Geometry check sheet. Reference: the model listing, model coordinates, mm. Give positions to 0.01 mm unless a question says otherwise; leave off trailing zeros. Loops run counter-clockwise (first coordinate to the right, second up) from the corner with the lowest first, then second, coordinate; pieces in that order, holes last.
1. Release check for a two-part mould opening along Z. For faces 1 (the flat face through (-1, -2, -6)), 2 (the flat face through (12.167, -0.986, 53.67)), 3 (the flat face through (-12.12, -0.99, 53.75)), 4 (the cylindrical face through (34.82, -0.99, 40.02)) record: +Z half, -Z half, draft (parallel to the pull), parting line (faces both ways), or undercut.
2. Cross-section at C-C, the plane z = 15. Record the cut outline in (x, y), plus the area to 3 significant figures.
3. Material ranges on L1, parallel to Z at x = 0, y = -1.05; L2, parallel to X at y = -1.1, z = -0.5; L3, parallel to X at y = -0.35, z = -10, recorded low to high.
4. Go/stop test with flat-tipped pins: pin 1 Ø0.6 at (x, y) = (-67, -1.5) entering from -Z; pin 2 Ø1 at (x, y) = (-25, -0.5) entering from +Z. Record where each tip stops, or that it passes through.
5. Cross-section at A-A, the plane y = -1.3. Record the cut outline in (x, z).
6. Cross-section at B-B, the plane x = 14. Record the cut outline in (y, z).
from build123d import *

# Parameters (mm, degrees)
F1_DEPTH = 2


# Not quite as in the source:
# - a feature names something its author has since deleted; it is built from what else it names


with BuildPart() as f1:
    # F0 (on Front) → F1 (new body)
    with BuildSketch(Plane.XZ):
        with BuildLine():
            ThreePointArc((19.4604751144, -49.3491610835), (25.0909627965, -46.7385641336), (30.3780152375, -43.4882280802))
            ThreePointArc((30.3780152375, -43.4882280802), (47.0400422182, -24.5210974354), (53.0476181494, 0))
            Line((53.0476181494, 0), (-53.0476181494, 0))
            ThreePointArc((-53.0476181494, 0), (-43.8541995948, -29.8472606654), (-19.4604751144, -49.3491610835))
            ThreePointArc((-19.4604751144, -49.3491610835), (-6.4361640705, -14.8511496358), (23.054123582, -36.9886383414))
            ThreePointArc((23.054123582, -36.9886383414), (22.1374887057, -43.4248024119), (19.4604751144, -49.3491610835))
        make_face()
        with BuildLine():
            Line((-53.0476181494, 0), (53.0476181494, 0))
            ThreePointArc((53.0476181494, 0), (51.7146557328, 11.817113597), (47.7827569309, 23.0403544115))
            Line((47.7827569309, 23.0403544115), (15.6281781272, 50.6932918615))
            ThreePointArc((15.6281781272, 50.6932918615), (9.002371997, 52.2781702984), (2.2280864718, 53.0008058618))
            ThreePointArc((2.2280864718, 53.0008058618), (0, 52.7800319348), (-2.2280864718, 53.0008058618))
            ThreePointArc((-2.2280864718, 53.0008058618), (-9.0528372764, 52.2694550246), (-15.7260278086, 50.6630224196))
            Line((-15.7260278086, 50.6630224196), (-47.6465335474, 23.3207553961))
            ThreePointArc((-47.6465335474, 23.3207553961), (-51.6797102792, 11.9690156981), (-53.0476181494, 0))
        make_face()
        with BuildLine():
            ThreePointArc((47.7827569309, 23.0403544115), (51.7146557328, 11.817113597), (53.0476181494, 0))
            Line((53.0476181494, 0), (74.573867023, 0))
            Line((74.573867023, 0), (47.7827569309, 23.0403544115))
        make_face()
        with BuildLine():
            ThreePointArc((-19.4604751144, -49.3491610835), (0, -60.0427619235), (19.4604751144, -49.3491610835))
            ThreePointArc((19.4604751144, -49.3491610835), (0, -53.0476181494), (-19.4604751144, -49.3491610835))
        make_face()
        with BuildLine():
            ThreePointArc((-19.4604751144, -49.3491610835), (0, -53.0476181494), (19.4604751144, -49.3491610835))
            ThreePointArc((19.4604751144, -49.3491610835), (22.1374887057, -43.4248024119), (23.054123582, -36.9886383414))
            ThreePointArc((23.054123582, -36.9886383414), (-6.4361640705, -14.8511496358), (-19.4604751144, -49.3491610835))
        make_face()
        with BuildLine():
            Line((15.6281781272, 50.6932918615), (47.7827569309, 23.0403544115))
            ThreePointArc((47.7827569309, 23.0403544115), (34.5891299202, 40.2199189791), (15.6281781272, 50.6932918615))
        make_face()
        with BuildLine():
            Line((-74.8721584678, 0), (-53.0476181494, 0))
            ThreePointArc((-53.0476181494, 0), (-51.6797102792, 11.9690156981), (-47.6465335474, 23.3207553961))
            Line((-47.6465335474, 23.3207553961), (-74.8721584678, 0))
        make_face()
        with BuildLine():
            ThreePointArc((2.2280864718, 53.0008058618), (9.002371997, 52.2781702984), (15.6281781272, 50.6932918615))
            Line((15.6281781272, 50.6932918615), (8.6080503312, 56.7306016959))
            ThreePointArc((8.6080503312, 56.7306016959), (5.730035728, 54.3320712807), (2.2280864718, 53.0008058618))
        make_face()
        with BuildLine():
            ThreePointArc((-15.7260278086, 50.6630224196), (-34.5097127589, 40.2880815704), (-47.6465335474, 23.3207553961))
            Line((-47.6465335474, 23.3207553961), (-15.7260278086, 50.6630224196))
        make_face()
        with BuildLine():
            ThreePointArc((-2.2280864718, 53.0008058618), (0, 53.0476181494), (2.2280864718, 53.0008058618))
            ThreePointArc((2.2280864718, 53.0008058618), (5.730035728, 54.3320712807), (8.6080503312, 56.7306016959))
            Line((8.6080503312, 56.7306016959), (0, 64.1335248947))
            Line((0, 64.1335248947), (-8.6226387996, 56.7475989187))
            ThreePointArc((-8.6226387996, 56.7475989187), (-5.7397015847, 54.3377284437), (-2.2280864718, 53.0008058618))
        make_face()
        with BuildLine():
            Line((0, 64.1335248947), (8.6080503312, 56.7306016959))
            ThreePointArc((8.6080503312, 56.7306016959), (10.6450279761, 60.1857176833), (11.3534929599, 64.1335248947))
            ThreePointArc((11.3534929599, 64.1335248947), (-3.9373045021, 74.7824420063), (-8.6226387996, 56.7475989187))
            Line((-8.6226387996, 56.7475989187), (0, 64.1335248947))
        make_face()
        with BuildLine():
            Line((-8.6226387996, 56.7475989187), (-15.7260278086, 50.6630224196))
            ThreePointArc((-15.7260278086, 50.6630224196), (-9.0528372764, 52.2694550246), (-2.2280864718, 53.0008058618))
            ThreePointArc((-2.2280864718, 53.0008058618), (-5.7397015847, 54.3377284437), (-8.6226387996, 56.7475989187))
        make_face()
    extrude(amount=F1_DEPTH)


solid = f1.part
Result:
1. face 1: draft
1. face 2: undercut
1. face 3: undercut
1. face 4: +Z half
2. outline: (-57.36, -2) - (57.13, -2) - (57.13, 0) - (-57.36, 0) - close
2. area: 229 mm2
3. L1: z = -60.04 to 52.78, 53.05 to 75.49
3. L2: x = -53.05 to 53.05
3. L3: x = -52.1 to 52.1
4. pin 1: stops at z = 0
4. pin 2: stops at z = 47.05
5. outline: (-74.87, 0) - (-53.05, 0) arc R53.05 ccw to (-19.46, -49.35) arc R23.05 ccw to (19.46, -49.35) arc R53.05 ccw to (53.05, 0) - (74.57, 0) - (47.78, 23.04) arc R53.05 ccw to (15.63, 50.69) - (8.61, 56.73) arc R11.35 ccw (long way) to (-8.62, 56.75) - (-15.73, 50.66) arc R53.05 ccw to (-47.65, 23.32) - close; hole (-2.23, 53) arc R11.35 ccw to (2.23, 53) arc R53.05 ccw to start
6. outline: (-2, -55.31) - (0, -55.31) - (0, 52.09) - (-2, 52.09) - close
